Geometry: final body of the model. Coordinates: model frame, mm. A direction names the side the tool comes from. Give positions to 0.01 mm unless a question says otherwise; leave off trailing zeros. Order: outer loops, then holes, each group sorted by start corner. A loop starts at its lowest first (then second) coordinate and runs counter-clockwise, first axis right, second up. Notation, with made-up numbers: (39.25, 19) - (87.25, 19) arc R13 ccw to (87.25, 23) - close; hole circle Ø7 at (2, -27). An arc over 180 degrees is marked (long way). Put each result on its own line as item: value. Start each with the question number.
1. Mould query, pull axis Z, two halves, no side actions, for faces 1 (the cylindrical face through (0, 0.5, -5.2)), 2 (the cylindrical face through (-1.38, 1.97, 6.2)), 3 (the flat face through (-2, 0, 4)), 4 (the cylindrical face through (4.2, 0.5, -0.1)). Classes: pulls with the +Z half, pulls with the -Z half, needs draft (parallel to the pull), parting line crosses it, or undercut.
2. Section C-C on x = 0. Return the cut outline in (y, z), plus the area to 3 significant figures.
3. Section B-B on y = 0.5. Return the cut outline in (x, z), plus the area to 3 significant figures.
4. Section D-D on y = 2.55. Return the cut outline in (x, z), plus the area to 3 significant figures.
5. Ray query, line 1 along Z through (x, y) = (0, 0.5); line 2 along Y through (x, z) = (-1.25, -3.5); line 3 along X through (y, z) = (0.3, 4.2). Return the intervals inside material, ascending. Write a range as from..to.
6. Set-up query: faces 5 (the flat face through (0, 1, 0)), 6 (the flat face through (0, 4, 0)). Return all of +Z, -Z, +X, -X, +Y, -Y with unobstructed straight access to the full face (end or side cutting, diameter ignored); none if empty.
7. Section A-A on z = 0. Return the cut outline in (x, y), plus the area to 3 significant figures.
8. First-contact query: P1, Ø1.5, axis at y = 3, z = 1.5, coming from the -X side; P2, Ø1, axis at y = 1, z = 2.5, coming from the +X side. Flat tips, straight axial feed; report the tip coordinate or a pass-through.
from build123d import *

# Parameters (mm, degrees)
SKETCH1_R           = 6.35
BOSS_EXTRUDE1_DEPTH = 4
SKETCH2_R           = 1
CUT_EXTRUDE2_DEPTH  = 1
SKETCH2_3_R         = 4.2
SKETCH2_3_R_2       = 1
CUT_EXTRUDE3_DEPTH  = 1


with BuildPart() as part:
    # Sketch1 → Boss-Extrude1 (new body)
    with BuildSketch(Plane(origin=(0, 0, 0), x_dir=(1, 0, 0), z_dir=(0, 1, 0))):
        Circle(SKETCH1_R)
    extrude(amount=BOSS_EXTRUDE1_DEPTH)

    # Sketch2 → Cut-Extrude2 (cut)
    with BuildSketch(Plane.XZ):
        with Locations((0, -4.2)):
            Circle(SKETCH2_R)
    extrude(amount=-CUT_EXTRUDE2_DEPTH, mode=Mode.SUBTRACT)

    # Sketch2<3> → Cut-Extrude3 (cut)
    with BuildSketch(Plane.XZ):
        Circle(SKETCH2_3_R)
        with Locations((0, 4.2)):
            Circle(SKETCH2_3_R_2)
    extrude(amount=-CUT_EXTRUDE3_DEPTH, mode=Mode.SUBTRACT)


solid = part.part
Resolved:
1. face 1: undercut
1. face 2: parting line crosses it
1. face 3: needs draft
1. face 4: undercut
2. outline: (0, -6.35) - (4, -6.35) - (4, 6.35) - (0, 6.35) - (0, 5.2) - (1, 5.2) - (1, -5.2) - (0, -5.2) - close
2. area: 40.4 mm^2
3. outline: circle Ø12.7 at (0, 0); hole (-0.99, -4.08) arc R1 ccw (long way) to (0.99, -4.08) arc R4.2 ccw to (0.99, 4.08) arc R1 ccw (long way) to (-0.99, 4.08) arc R4.2 ccw to start
3. area: 68.0 mm^2
4. outline: circle Ø12.7 at (0, 0)
4. area: 127 mm^2
5. line 1: -6.35..-5.2, 5.2..6.35
5. line 2: 1..4
5. line 3: -4.76..-1, 1..4.76
6. face 5: -Y
6. face 6: +Z, -Z, +X, -X, +Y
7. outline: (-6.35, 0) - (-4.2, 0) - (-4.2, 1) - (4.2, 1) - (4.2, 0) - (6.35, 0) - (6.35, 4) - (-6.35, 4) - close
7. area: 42.4 mm^2
8. P1: x = -6.31
8. P2: x = 6.03
